Can you work these out from the model? Positions are in its coordinate system, mm. A direction names the side the tool comes from. Give positions to 0.01 mm unless a question says otherwise; leave off trailing zeros. Loops run counter-clockwise (first coordinate to the right, second up) from the corner with the lowest first, then second, coordinate; pieces in that order, holes last. Notation, with made-up numbers: (31.5, 36) -> (35.5, 36) arc R19 cw to (35.5, 72) -> close; hole circle Ø9 at (12, 30.5). An arc over 180 degrees is marked (long way). Return JSON: item names as keys, results as strings. Group by question number.
Q1. Thinking about a two-plate mould opening in Z: for faces 1 (the flat face through (-4, 125, 762)), 2 (the flat face through (4, 0, 11)), 3 (the flat face through (-3, 25.4, -10)), which applies, pulls with the +Z half, pulls with the -Z half, needs draft (parallel to the pull), parting line crosses it, or undercut?
Q2. Which directions (+Z, -Z, +X, -X, +Y, -Y) give clear straight access to the entire face, cutting with the end or side of a thin tool? Please do faces 4 (the cylindrical face through (-13.65, 72.22, -749.48)), 5 (the flat face through (246, 254, 229)), 6 (the flat face through (228.6, 141, 10)).
Q3. I need wall thicknesses on line 1 along Y through (x, z) = (0, -752); line 2 along Z through (x, y) = (37.5, 196); line 3 along X through (y, z) = (50.8, -745.5). Which ranges of each line are inside material? Lowest first, please. Write a range as [from, to].
Q4. Suppose I cut it at B-B, the plane x = -193. Please give me the cut outline in (y, z), and give its area (3 significant figures).
Q5. Suppose I cut it at C-C, the plane z = -364.5. Please give me the cut outline in (x, y), and give its area (3 significant figures).
Q6. Will this pin go through, and if not, where does the flat tip stop? pin 1 (3 mm diameter, centred on x = -87.5, z = -554, fed in from +Y).
Q7. Suppose I cut it at D-D, the plane y = 192. Please give me the cut outline in (x, z).
Q8. Suppose I cut it at A-A, the plane y = 50.8. Please give me the cut outline in (x, z).
Autodesk Inventor part; units mm, degrees
ref_plane "YZ Plane" through (0, 0, 0) normal (1, 0, 0) x (0, 1, 0)
ref_plane "XZ Plane" through (0, 0, 0) normal (0, 1, 0) x (-1, 0, 0)
ref_plane "XY Plane" through (0, 0, 0) normal (0, 0, 1) x (1, 0, 0)
sketch "Sketch1" plane through (0, 0, 0) normal (0, 1, 0) x (-1, 0, 0)
  line L0 (254, 762) -> (-254, 762)
  line L1 (-254, 762) -> (-254, -762)
  line L2 (-254, -762) -> (254, -762)
  line L3 (254, -762) -> (254, 762)
  line L4 (254, 762) -> (-254, -762) construction
  line L5 (-254, 762) -> (254, -762) construction
  point P0 (0, 0)
  dimension "d0" = 508
  dimension "d1" = 1524
extrude "Extrusion1" add sketch "Sketch1" along normal blind 254
sketch "Sketch2" plane through (0, 254, 0) normal (0, 1, 0) x (1, 0, 0)
  line L0 (-254, -762) -> (254, -762)
  line L1 (254, 762) -> (-254, 762)
  line L2 (-254, 762) -> (-254, -762)
  line L3 (-254, -762) -> (254, -762)
  line L4 (254, -762) -> (254, 762)
  line L5 (254, 762) -> (-254, -762) construction
  line L6 (-254, 762) -> (254, -762) construction
  line L7 (0, -762) -> (0, -736.6)
  line L8 (-254, 762) -> (-254, -762)
  line L9 (-254, 0) -> (-228.6, 0)
  line L10 (228.6, 736.6) -> (-228.6, 736.6)
  line L11 (-228.6, 736.6) -> (-228.6, -736.6)
  line L12 (-228.6, -736.6) -> (228.6, -736.6)
  line L13 (228.6, -736.6) -> (228.6, 736.6)
  line L14 (228.6, 736.6) -> (-228.6, -736.6) construction
  line L15 (-228.6, 736.6) -> (228.6, -736.6) construction
  point P0 (0, 0)
  dimension "d4" = 25.4
  dimension "d5" = 25.4
extrude "Extrusion2" cut sketch "Sketch2" against normal blind 228.6 contours L12 L11 L10 L13
sketch "Sketch3" plane through (254, 0, -762) normal (0, 0, -1) x (-1, 0, 0)
  line L0 (25.4, 254) -> (482.6, 254)
  line L1 (254, 254) -> (254, 50.8) construction
  circle A0 centre (254, 50.8) radius 25.4
  point P0 (254, 0)
  dimension "d8" = 203.2
  dimension "d9" = 50.8
extrude "Extrusion3" cut sketch "Sketch3" against normal blind 228.6
properties part number "Trough"
Ans:
{
 "1": {"face 1": "pulls with the +Z half", "face 2": "needs draft", "face 3": "undercut"},
 "2": {"face 4": "-Z", "face 5": "+Z, -Z, +X, -X, +Y", "face 6": "+Y"},
 "3": {"line 1": "y = [0, 25.4], [76.2, 254]", "line 2": "z = [-762, -736.6], [736.6, 762]", "line 3": "x = [-254, -25.4], [25.4, 254]"},
 "4": {"outline": "(0, -762) -> (254, -762) -> (254, -736.6) -> (25.4, -736.6) -> (25.4, 736.6) -> (254, 736.6) -> (254, 762) -> (0, 762) -> close", "area": "50,300 mm^2"},
 "5": {"outline": "(-254, 0) -> (254, 0) -> (254, 254) -> (228.6, 254) -> (228.6, 25.4) -> (-228.6, 25.4) -> (-228.6, 254) -> (-254, 254) -> close", "area": "24,500 mm^2"},
 "6": {"pin 1": "stops at y = 25.4"},
 "7": {"outline": "(-254, -762) -> (254, -762) -> (254, 762) -> (-254, 762) -> close; hole (-228.6, -736.6) -> (228.6, -736.6) -> (228.6, 736.6) -> (-228.6, 736.6) -> close"},
 "8": {"outline": "(-254, -762) -> (-25.4, -762) -> (-25.4, -736.6) -> (-228.6, -736.6) -> (-228.6, 736.6) -> (228.6, 736.6) -> (228.6, -736.6) -> (25.4, -736.6) -> (25.4, -762) -> (254, -762) -> (254, 762) -> (-254, 762) -> close"}
}
